Design review of the part shown in the three views and the two pictorial views. Dimensions are in mm from the part's minimum x, y and z. Coordinates: 2 decimals unless noted, no trailing zeros. Write each loop counter-clockwise with the first axis right and the second up, starting at its lowest first coordinate (ties: lowest second). Pieces come first, ordered by that corner, then holes. Notation, with made-up numbers: (46, 48.25) - (54, 48.25) arc R29 cw to (54, 78.25) - close; hole circle Ø11 at (51.5, -18.75). An arc over 180 degrees is marked (long way). Return JSON: item names as keys, results as strings. Group by question number.
(1) We need section C-C on y = 6. State the section outline as (x, z) points.
(2) We need section A-A on z = 5. State the section outline as (x, y) points.
(3) We need section D-D on z = 8. State the section outline as (x, y) points, then the cut area to 3 significant figures.
(4) We need section B-B on x = 6. State the section outline as (y, z) points.
(5) For pin 1 Ø2.5 at (x, z) = (6, 5) entering from -Y; pin 2 Ø4.5 at (x, y) = (6, 6) entering from -Z; pin 3 Ø1.5 at (y, z) = (10.5, 14.5) entering from -X, all flat-tipped, find the tip position at first contact; note any pin that passes through.
(6) Draft analysis for pull direction Y (two halves, no side actions). For the marked faces 1, 2 and 3, state which applies: released by +Y, released by -Y, zero draft, split by the parting line, or undercut.
(7) To check wall thickness, follow L1, parallel to Z at x = 6, y = 10.5; L2, parallel to X at y = 9.75, z = 5.5; L3, parallel to X at y = 5.5, z = 2.5. State the ranges of each line that lie inside material, in increasing order. Write a range as from..to.
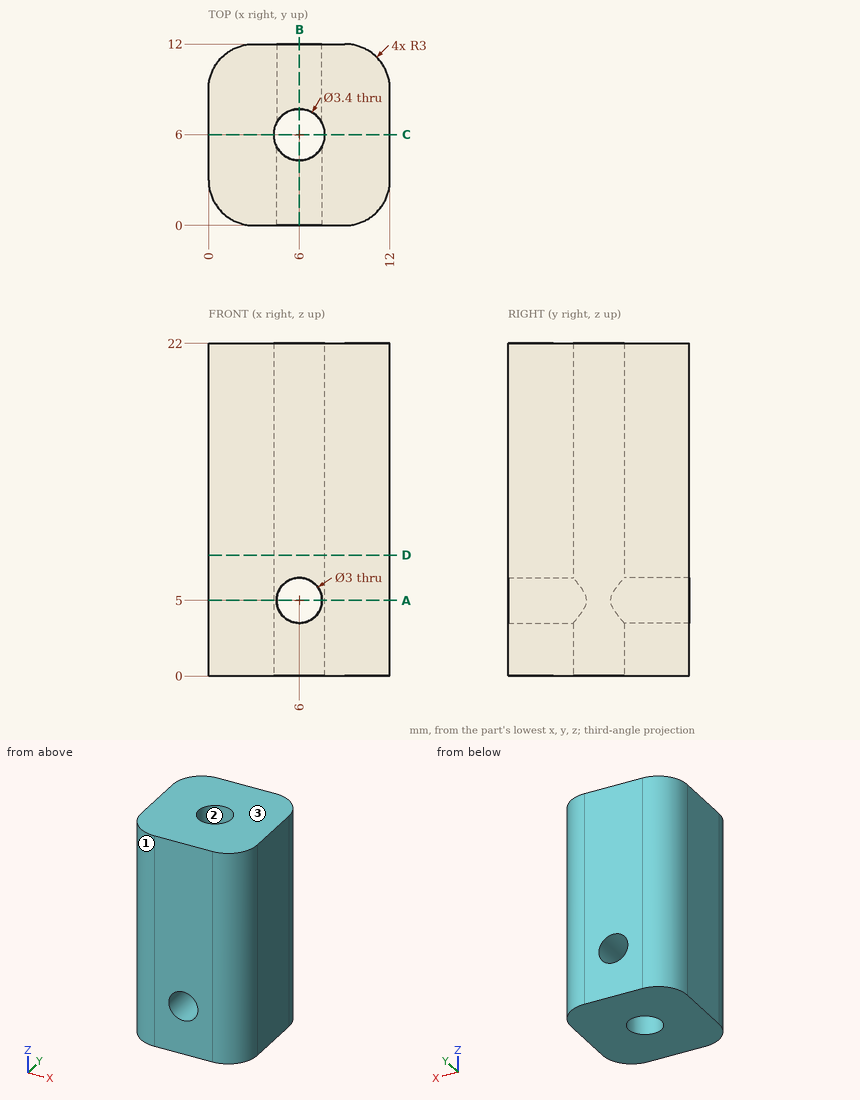
Ans:
{
 "1": {"outline": "(0, 0) - (4.3, 0) - (4.3, 22) - (0, 22) - close; (7.7, 0) - (12, 0) - (12, 22) - (7.7, 22) - close"},
 "2": {"outline": "(0, 3) arc R3 ccw to (3, 0) - (4.5, 0) - (4.5, 5.2) arc R1.7 cw to (4.5, 6.8) - (4.5, 12) - (3, 12) arc R3 ccw to (0, 9) - close; (7.5, 0) - (9, 0) arc R3 ccw to (12, 3) - (12, 9) arc R3 ccw to (9, 12) - (7.5, 12) - (7.5, 6.8) arc R1.7 cw to (7.5, 5.2) - close"},
 "3": {"outline": "(0, 3) arc R3 ccw to (3, 0) - (9, 0) arc R3 ccw to (12, 3) - (12, 9) arc R3 ccw to (9, 12) - (3, 12) arc R3 ccw to (0, 9) - close; hole circle Ø3.4 at (6, 6)", "area": "127 mm²"},
 "4": {"outline": "(0, 0) - (4.3, 0) - (4.3, 3.5) - (0, 3.5) - close; (0, 6.5) - (4.3, 6.5) - (4.3, 22) - (0, 22) - close; (7.7, 0) - (12, 0) - (12, 3.5) - (7.7, 3.5) - close; (7.7, 6.5) - (12, 6.5) - (12, 22) - (7.7, 22) - close"},
 "5": {"pin 1": "through", "pin 2": "z = 0", "pin 3": "x = 0.1"},
 "6": {"face 1": "released by -Y", "face 2": "undercut", "face 3": "zero draft"},
 "7": {"L1": "0..3.5, 6.5..22", "L2": "0.1..4.59, 7.41..11.9", "L3": "0..4.38, 7.62..12"}
}
